```python
from build123d import *

# Parameters (mm, degrees)
F1_DEPTH = 10
F2_R     = 2.5
F3_DEPTH = 26.918743
F4_W     = 3
F4_H     = 3
F5_DEPTH = 5


with BuildPart() as f1:
    # F0 (on Right) → F1 (new body, symmetric)
    with BuildSketch(Plane.YZ):
        Polygon((9.460487, 8.417743), (9.460487, 13.917743), (29.460487, 13.917743), (56.460487, 23.917743), (156.460487, 23.917743), (156.460487, 26.917743), (56.460487, 26.917743), (29.460487, 16.917743), (6.460487, 16.917743), (6.460487, 8.417743), align=None)
    extrude(amount=F1_DEPTH, both=True)

    # F2 (on Top) → F3 (cut, through all)
    with BuildSketch(Plane.XY):
        with Locations((0, 19.460487)):
            Circle(F2_R)
    extrude(amount=F3_DEPTH, mode=Mode.SUBTRACT)

    # F4 (on face) → F5 (join)
    with BuildSketch(Plane(origin=(0, 0, 8.417743), x_dir=(1, 0, 0), z_dir=(0, 0, -1))):
        with Locations((0, -7.960487)):
            Rectangle(F4_W, F4_H)
    extrude(amount=F5_DEPTH)


solid = f1.part
```
Geometry: final body of the model. Coordinates: model frame, mm. A direction names the side the tool comes from. Give positions to 0.01 mm unless a question says otherwise; leave off trailing zeros. Write each loop counter-clockwise with the first axis right and the second up, starting at its lowest first coordinate (ties: lowest second). Pieces come first, ordered by that corner, then holes.
1. Section query A-A, the plane x = 0. Return loops of the section in (y, z), then the cut area to 4 significant figures.
2. Section query C-C, the plane y = 37. Return loops of the section in (x, z), then the cut area to 3 significant figures.
3. Reachability of faces 1 (the flat face through (2.4, 18.1, 16.918)), 2 (the flat face through (-1.5, 8, 6)), 3 (the flat face through (1.5, 8, 6)) from +Z, -Z, +X, -X, +Y, -Y: full face, straight path, thin tool, end or side. Return the list, or none.
4. Line query: probe 1 along Y at (x, z) = (-4.25, 12.5); probe 2 along Z at (x, y) = (-3, 75.5); probe 3 along Z at (x, y) = (-5.75, 19). Output: solid intervals per line, ascending.
5. Section query B-B, the plane z = 5.75. Return loops of the section in (x, y).
6. Pin query (flat end, axial travel): P1, Ø2, axis at x = -1.5, y = 49.5, coming from the -Z side; P2, Ø8, axis at x = -8, y = 86.5, coming from the -Z side; P3, Ø0.9, axis at y = 7, z = 7, coming from the -X side. Return the tip coordinate at first contact, or that it passes through.
Computed:
1. outline: (6.46, 3.42) - (9.46, 3.42) - (9.46, 13.92) - (16.96, 13.92) - (16.96, 16.92) - (6.46, 16.92) - close; (21.96, 13.92) - (29.46, 13.92) - (56.46, 23.92) - (156.46, 23.92) - (156.46, 26.92) - (56.46, 26.92) - (29.46, 16.92) - (21.96, 16.92) - close
1. area: 466.5 mm2
2. outline: (-10, 16.71) - (10, 16.71) - (10, 19.71) - (-10, 19.71) - close
2. area: 60.0 mm2
3. face 1: +Z, +X, -X, -Y
3. face 2: -Z, -X, +Y, -Y
3. face 3: -Z, +X, +Y, -Y
4. probe 1: y = 6.46 to 9.46
4. probe 2: z = 23.92 to 26.92
4. probe 3: z = 13.92 to 16.92
5. outline: (-1.5, 6.46) - (1.5, 6.46) - (1.5, 9.46) - (-1.5, 9.46) - close
6. P1: stops at z = 20.97
6. P2: stops at z = 23.92
6. P3: stops at x = -1.5
